Can you work these out from the model? Positions are in its coordinate system, mm. Face numbers are marked on the shaded views. A direction names the side the tool comes from. Coordinates: 2 decimals unless noted, no trailing zeros. Order: outer loops, then holes, each group sorted by start corner. A loop starts at its lowest first (then second) coordinate and runs counter-clockwise, first axis right, second up. Notation, with made-up numbers: (84.25, -39) -> (117.25, -39) arc R31 ccw to (117.25, -2) -> close; hole circle Ø8 at (62.5, 60.5). An arc over 180 degrees is marked (long way). Write item = value, one per line.
```python
from build123d import *

# Parameters (mm, degrees)
SKETCH1_W           = 3
SKETCH1_H           = 15
BOSS_EXTRUDE1_DEPTH = 10
CUT_EXTRUDE1_DEPTH  = 60.42432162


with BuildPart() as part:
    # Sketch1 → Boss-Extrude1 (new body)
    with BuildSketch(Plane(origin=(0, 0, 0), x_dir=(1, 0, 0), z_dir=(0, 1, 0))):
        Polygon((19.5, -19.5), (19.5, 19.5), (-19.5, 19.5), (-19.5, -19.5), (-19.5, -22.5), (-22.5, -22.5), (-22.5, 22.5), (22.5, 22.5), (22.5, -22.5), (19.5, -22.5), align=None)
        with Locations((-21, -30)):
            Rectangle(SKETCH1_W, SKETCH1_H)
        with Locations((21, -30)):
            Rectangle(SKETCH1_W, SKETCH1_H)
    extrude(amount=BOSS_EXTRUDE1_DEPTH)

    # Sketch3 → Cut-Extrude1 (cut, through all)
    with BuildSketch(Plane(origin=(22.5, 0, 0), x_dir=(0, 0, -1), z_dir=(1, 0, 0))):
        Polygon((-32.5, 8), (-35.5, 5), (-32.5, 2), (-29.5, 5), align=None)
    extrude(amount=-CUT_EXTRUDE1_DEPTH, mode=Mode.SUBTRACT)


solid = part.part
```
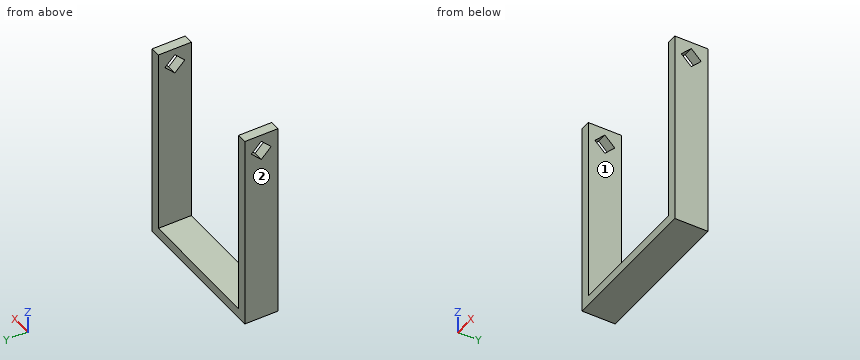
Item 1: For the marked faces 1 and 2, which set-ups out of +Z, -Z, +X, -X, +Y, -Y let a thin tool reach every point of the face, with its end or its side?
A:
face_1 = +Z, +Y, -Y
face_2 = +Z, -Z, -X, +Y, -Y
Item 2: I want a section at A-A, the plane z = 11.5. Please give me the cut outline in (x, y), plus the area to 3 significant figures.
A:
outline = (-22.5, 0) -> (-19.5, 0) -> (-19.5, 10) -> (-22.5, 10) -> close; (19.5, 0) -> (22.5, 0) -> (22.5, 10) -> (19.5, 10) -> close
area = 60.0 mm2
Item 3: I want a section at C-C, the plane z = 31. Please give me the cut outline in (x, y), plus the area to 3 significant figures.
A:
outline = (-22.5, 0) -> (-19.5, 0) -> (-19.5, 3.5) -> (-22.5, 3.5) -> close; (-22.5, 6.5) -> (-19.5, 6.5) -> (-19.5, 10) -> (-22.5, 10) -> close; (19.5, 0) -> (22.5, 0) -> (22.5, 3.5) -> (19.5, 3.5) -> close; (19.5, 6.5) -> (22.5, 6.5) -> (22.5, 10) -> (19.5, 10) -> close
area = 42.0 mm2
Item 4: I want a section at D-D, the plane y = 9.25. Please give me the cut outline in (x, z), plus the area to 3 significant figures.
A:
outline = (-22.5, -22.5) -> (22.5, -22.5) -> (22.5, 37.5) -> (19.5, 37.5) -> (19.5, -19.5) -> (-19.5, -19.5) -> (-19.5, 37.5) -> (-22.5, 37.5) -> close
area = 477 mm2
Item 5: I want a section at B-B, the plane y = 4. Please give me the cut outline in (x, z).
A:
outline = (-22.5, -22.5) -> (22.5, -22.5) -> (22.5, 30.5) -> (19.5, 30.5) -> (19.5, -19.5) -> (-19.5, -19.5) -> (-19.5, 30.5) -> (-22.5, 30.5) -> close; (-22.5, 34.5) -> (-19.5, 34.5) -> (-19.5, 37.5) -> (-22.5, 37.5) -> close; (19.5, 34.5) -> (22.5, 34.5) -> (22.5, 37.5) -> (19.5, 37.5) -> close
Item 6: I'm going to push flat-ended pins straight in: P1, Ø3, axis at x = 15.5, y = 4, coming from the +Z side; P2, Ø6, axis at x = 5.5, z = -16, coming from the -Y side. Where does each tip first touch, or does it pass through?
A:
P1 = -19.5
P2 = through
Item 7: If I drill on probe 1 along X at (y, z) = (3.5, 5.5); probe 2 along Z at (x, y) = (4, 8), over which ranges is the centre line in solid material (lowest first)?
A:
probe_1 = -22.5 to -19.5, 19.5 to 22.5
probe_2 = -22.5 to -19.5
